from build123d import *

# Parameters (mm, degrees)
BOSS_EXTRUDE1_DEPTH = 12.5
BOSS_EXTRUDE2_DEPTH = 12
SKETCH2_W           = 4.747951262
SKETCH2_H           = 6.647569448
SKETCH2_W_2         = 4.499129778
BOSS_EXTRUDE3_DEPTH = 10


with BuildPart() as part:
    # Sketch1 → Boss-Extrude1 (new, symmetric)
    with BuildSketch(Plane(origin=(0, 0, 0), x_dir=(0, 0, -1), z_dir=(1, 0, 0))):
        with BuildLine():
            Line((5, 0), (-5, 0))
            Line((-5, 0), (-5, 3))
            Line((-5, 3), (-5, 9))
            ThreePointArc((-5, 9), (0, 4), (5, 9))
            Line((5, 9), (5, 3))
            Line((5, 3), (5, 0))
        make_face()
    extrude(amount=BOSS_EXTRUDE1_DEPTH, both=True)

    # Sketch1<5> → Boss-Extrude2 (add, symmetric)
    with BuildSketch(Plane(origin=(0, 0, 0), x_dir=(0, 0, -1), z_dir=(1, 0, 0))):
        with BuildLine():
            ThreePointArc((-5, 9), (-3.535533906, 5.464466094), (0, 4))
            ThreePointArc((0, 4), (3.535533906, 5.464466094), (5, 9))
            ThreePointArc((5, 9), (0, 14), (-5, 9))
        make_face()
    extrude(amount=BOSS_EXTRUDE2_DEPTH, both=True)

    # Sketch2 → Boss-Extrude3 (add)
    with BuildSketch(Plane.XY.offset(5)):
        with Locations((-9.073174039, 9)):
            Rectangle(SKETCH2_W, SKETCH2_H)
        with Locations((7.477413935, 9)):
            Rectangle(SKETCH2_W_2, SKETCH2_H)
    extrude(amount=-BOSS_EXTRUDE3_DEPTH)


solid = part.part
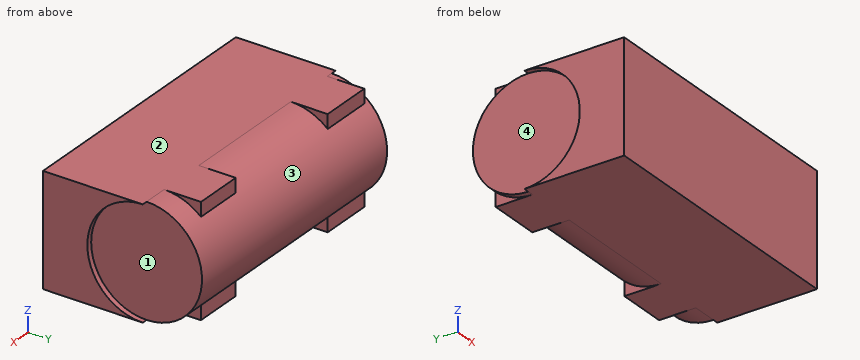
Work out the finished part from the listing and answer in its coordinate system (mm). Face numbers are marked on the shaded views. A direction names the side the tool comes from. Give positions to 0.01 mm unless a question says otherwise; leave off trailing zeros. Write each loop counter-clockwise with the first axis right and the second up, starting at its lowest first coordinate (ties: lowest second). Pieces come first, ordered by that corner, then holes. Notation, with made-up numbers: (-7.5, 86.25) - (33.5, 86.25) arc R6 cw to (33.5, 93.25) - close; hole circle Ø11 at (-20, 85.5). An arc over 180 degrees is marked (long way). One line per item, written item: value. Start each with the question number.
1. Find section A-A (z = 4). Write down the section's boundary in (x, y), then the cut area to 3 significant figures.
2. For the marked faces 1, 2, 3 and 4, determine the directions among +Z, -Z, +X, -X, +Y, -Y from which every point of the face is accessible in a straight line to the end or side of a thin tool.
3. Find section C-C (x = 10.75). Write down the section's boundary in (y, z).
4. Consider probe 1 along X at (y, z) = (8, 0.75); probe 2 along Y at (x, z) = (-10, 4); probe 3 along Z at (x, y) = (-3, 10.5). Determine where each line is inside the solid, lowest interval first.
5. Find section B-B (y = 5). Write down the section's boundary in (x, z).
6. Given pin 1 (0.6 mm diameter, centred on x = -8.5, z = -4, fed in from +Y); pin 2 (1 mm diameter, centred on y = 10, z = 4.5, fed in from -X); pin 3 (1.5 mm diameter, centred on x = -0.5, z = -2, fed in from -Y); pin 4 (3 mm diameter, centred on x = -3.5, z = -4, fed in from +Y), each flat-ended and moving along its own axis, determine where each tip first touches the part or whether it passes through.
7. Find section D-D (z = 0). Write down the section's boundary in (x, y).
Geometry results:
1. outline: (-12.5, 0) - (12.5, 0) - (12.5, 6) - (12, 6) - (12, 12) - (9.73, 12) - (9.73, 12.32) - (5.23, 12.32) - (5.23, 12) - (-6.7, 12) - (-6.7, 12.32) - (-11.45, 12.32) - (-11.45, 12) - (-12, 12) - (-12, 6) - (-12.5, 6) - close
1. area: 297 mm2
2. face 1: +X, +Y
2. face 2: +Z, +X, -X, +Y, -Y
2. face 3: +Y
2. face 4: -X, +Y
3. outline: (0, -5) - (9, -5) arc R5 ccw to (9, 5) - (0, 5) - close
4. probe 1: -12 to 12
4. probe 2: 0 to 12.32
4. probe 3: -4.77 to 4.77
5. outline: (-12.5, -5) - (12.5, -5) - (12.5, -3) - (12, -3) - (12, 3) - (12.5, 3) - (12.5, 5) - (-12.5, 5) - (-12.5, 3) - (-12, 3) - (-12, -3) - (-12.5, -3) - close
6. pin 1: y = 12.36
6. pin 2: x = -12
6. pin 3: y = 0
6. pin 4: y = 13.33
7. outline: (-12.5, 0) - (12.5, 0) - (12.5, 4) - (12, 4) - (12, 14) - (-12, 14) - (-12, 4) - (-12.5, 4) - close
